```python
from build123d import *
from build123d.topology import SkipClean

# Parameters (mm, degrees)
SKETCH_1_W          = 101.5
SKETCH_1_H          = 91.5
SKETCH_1_W_2        = 98.5
SKETCH_1_H_2        = 88.5
EXTRUDE_1_DEPTH     = 21
SKETCH_2_W          = 101.5
SKETCH_2_H          = 91.5
SKETCH_2_R          = 1.5
SKETCH_2_W_2        = 31
SKETCH_2_H_2        = 31
EXTRUDE_2_DEPTH     = 1.5
SKETCH_3_R          = 1.75
CUT_EXTRUDE_1_DEPTH = 139.25881527
SKETCH_4_R          = 1.75
CUT_EXTRUDE_2_DEPTH = 139.25881527
FILLET_1_R          = 9
FILLET_2_R          = 10
FILLET_3_R          = 4
FILLET_4_R          = 5
EXTRUDE_START       = -3
SKETCH_5_R          = 47.5
SKETCH_5_R_2        = 1.5
SKETCH_5_W          = 45
SKETCH_5_H          = 46
EXTRUDE_3_DEPTH     = 3
SKETCH_6_R          = 47.5
SKETCH_6_R_2        = 43.5
EXTRUDE_4_DEPTH     = 13
SKETCH_7_R          = 49.25
SKETCH_7_R_2        = 43.5
EXTRUDE_5_DEPTH     = 9
SKETCH_8_R          = 44
SKETCH_8_R_2        = 5
CUT_EXTRUDE_3_DEPTH = 1.5
SKETCH_9_R          = 1.75
CUT_EXTRUDE_4_DEPTH = 141.599608819
SKETCH_10_R         = 3
CUT_EXTRUDE_5_DEPTH = 1.5


with BuildPart() as part:
    # 草图1 → 凸台-拉伸1 (new body)
    with BuildSketch(Plane(origin=(0, 0, 0), x_dir=(0, 0, -1), z_dir=(1, 0, 0))):
        with Locations((50.75, 45.75)):
            Rectangle(SKETCH_1_W, SKETCH_1_H)
        with Locations((50.75, 45.75)):
            Rectangle(SKETCH_1_W_2, SKETCH_1_H_2, mode=Mode.SUBTRACT)
    extrude(amount=EXTRUDE_1_DEPTH)

    # 草图2 → 凸台-拉伸2 (add)
    with BuildSketch(Plane.ZY):
        with Locations((-50.75, 45.75)):
            Rectangle(SKETCH_2_W, SKETCH_2_H)
        with Locations((-27.25, 71.5)):
            Circle(SKETCH_2_R, mode=Mode.SUBTRACT)
        with Locations((-22.25, 44.5)):
            Circle(SKETCH_2_R, mode=Mode.SUBTRACT)
        with Locations(Location((-79.25, 44.5, 0), (0, 0, 180))):
            Circle(SKETCH_2_R, mode=Mode.SUBTRACT)
        with Locations(Location((-74.25, 71.5, 0), (0, 0, 180))):
            Circle(SKETCH_2_R, mode=Mode.SUBTRACT)
        with Locations((-50.75, 45)):
            Rectangle(SKETCH_2_W_2, SKETCH_2_H_2, mode=Mode.SUBTRACT)
    extrude(amount=EXTRUDE_2_DEPTH)

    # 草图3 → 切除-拉伸1 (cut, through all)
    with BuildSketch(Plane.XY):
        with Locations((11, 45.75)):
            Circle(SKETCH_3_R)
    extrude(amount=-CUT_EXTRUDE_1_DEPTH, mode=Mode.SUBTRACT)

    # 草图4 → 切除-拉伸2 (cut, through all)
    with BuildSketch(Plane(origin=(0, 91.5, 0), x_dir=(1, 0, 0), z_dir=(0, 1, 0))):
        with Locations(Location((11, 16.75, 0), (0, 0, 270))):
            Circle(SKETCH_4_R)
        with Locations(Location((11, 84.75, 0), (0, 0, 90))):
            Circle(SKETCH_4_R)
    extrude(amount=-CUT_EXTRUDE_2_DEPTH, mode=Mode.SUBTRACT)

    # 圆角1
    fillet_1_edges = [part.edges().sort_by_distance(p)[0] for p in [
        (10.5, 90, -100),
        (10.5, 90, -1.5),
    ]]
    fillet(fillet_1_edges, radius=FILLET_1_R)

    # 圆角2
    fillet_2_edges = [part.edges().sort_by_distance(p)[0] for p in [
        (9.75, 91.5, 0),
        (9.75, 91.5, -101.5),
    ]]
    fillet(fillet_2_edges, radius=FILLET_2_R)

    # 圆角3
    fillet_3_edges = [part.edges().sort_by_distance(p)[0] for p in [
        (10.5, 1.5, -1.5),
        (10.5, 1.5, -100),
    ]]
    fillet(fillet_3_edges, radius=FILLET_3_R)

    # 圆角4
    fillet_4_edges = [part.edges().sort_by_distance(p)[0] for p in [
        (9.75, 0, -101.5),
        (9.75, 0, 0),
    ]]
    fillet(fillet_4_edges, radius=FILLET_4_R)

    # 草图5 → 凸台-拉伸3 (add)
    with BuildSketch(Plane.ZY.offset(1.5).offset(EXTRUDE_START)):
        with Locations((-50.75, 45.75)):
            Circle(SKETCH_5_R)
        with Locations((-27.25, 71.5)):
            Circle(SKETCH_5_R_2, mode=Mode.SUBTRACT)
        with Locations((-22.25, 44.5)):
            Circle(SKETCH_5_R_2, mode=Mode.SUBTRACT)
        with Locations(Location((-79.25, 44.5, 0), (0, 0, 180))):
            Circle(SKETCH_5_R_2, mode=Mode.SUBTRACT)
        with Locations(Location((-74.25, 71.5, 0), (0, 0, 180))):
            Circle(SKETCH_5_R_2, mode=Mode.SUBTRACT)
        with Locations((-50.75, 43)):
            Rectangle(SKETCH_5_W, SKETCH_5_H, mode=Mode.SUBTRACT)
    extrude(amount=EXTRUDE_3_DEPTH)

    # 草图6 → 凸台-拉伸4 (add)
    with BuildSketch(Plane(origin=(1.5, 0, 0), x_dir=(0, 0, -1), z_dir=(1, 0, 0))):
        with Locations(Location((50.75, 45.75, 0), (0, 0, 105.600995393))):
            Circle(SKETCH_6_R)
        with Locations((50.75, 45.75)):
            Circle(SKETCH_6_R_2, mode=Mode.SUBTRACT)
    extrude(amount=-EXTRUDE_4_DEPTH)

    # 草图7 → 凸台-拉伸5 (add)
    with BuildSketch(Plane.ZY.offset(11.5)):
        with Locations((-50.75, 45.75)):
            Circle(SKETCH_7_R)
        with Locations(Location((-50.75, 45.75, 0), (0, 0, 180))):
            Circle(SKETCH_7_R_2, mode=Mode.SUBTRACT)
    extrude(amount=EXTRUDE_5_DEPTH)

    # 草图8 → 切除-拉伸3 (cut)
    with BuildSketch(Plane(origin=(1.5, 0, 0), x_dir=(0, 0, -1), z_dir=(1, 0, 0))):
        with Locations((50.75, 45.75)):
            Circle(SKETCH_8_R)
        with Locations((74.25, 71.5)):
            Circle(SKETCH_8_R_2, mode=Mode.SUBTRACT)
        with Locations((79.25, 44.5)):
            Circle(SKETCH_8_R_2, mode=Mode.SUBTRACT)
        with Locations((22.25, 44.5)):
            Circle(SKETCH_8_R_2, mode=Mode.SUBTRACT)
        with Locations((27.25, 71.5)):
            Circle(SKETCH_8_R_2, mode=Mode.SUBTRACT)
    extrude(amount=-CUT_EXTRUDE_3_DEPTH, mode=Mode.SUBTRACT)

    # 草图9 → 切除-拉伸4 (cut, through all)
    with SkipClean():  # the faces are left unmerged after this step: merging them gives an invalid solid
        with BuildSketch(Plane.XY):
            with Locations((-6.5, 45.75)):
                Circle(SKETCH_9_R)
        extrude(amount=-CUT_EXTRUDE_4_DEPTH, mode=Mode.SUBTRACT)

    # 草图10 → 切除-拉伸5 (cut)
    with SkipClean():  # the faces are left unmerged after this step: merging them gives an invalid solid
        with BuildSketch(Plane.ZY.offset(1.5)):
            with Locations((-74.25, 71.5)):
                Circle(SKETCH_10_R)
            with Locations((-27.25, 71.5)):
                Circle(SKETCH_10_R)
            with Locations((-22.25, 44.5)):
                Circle(SKETCH_10_R)
            with Locations((-79.25, 44.5)):
                Circle(SKETCH_10_R)
        extrude(amount=-CUT_EXTRUDE_5_DEPTH, mode=Mode.SUBTRACT)


solid = part.part
```
Read the model definition and answer for the solid it produces. Units are mm, in the model's axes. A direction names the side the tool comes from. Give positions to 0.01 mm unless a question says otherwise; leave off trailing zeros. Write each loop counter-clockwise with the first axis right and the second up, starting at its lowest first coordinate (ties: lowest second). Pieces come first, ordered by that corner, then holes. Notation, with made-up numbers: (64.25, 5.5) -> (95.25, 5.5) arc R13 cw to (95.25, 30.5) -> close; hole circle Ø3 at (54, 6). An arc over 180 degrees is marked (long way). Answer as a JSON object with one key per item and string values.
1) Section A-A on z = -50.75 is taken. Write down the section's boundary in (x, y).
Findings below:
{"outline": "(-20.5, -3.5) -> (-11.5, -3.5) -> (-11.5, -1.75) -> (1.5, -1.75) -> (1.5, 0) -> (21, 0) -> (21, 1.5) -> (1.5, 1.5) -> (1.5, 1.75) -> (0, 1.75) -> (0, 29.5) -> (-1.5, 29.5) -> (-1.5, 2.25) -> (-20.5, 2.25) -> close; (-20.5, 89.25) -> (-1.5, 89.25) -> (-1.5, 60.5) -> (0, 60.5) -> (0, 89.75) -> (1.5, 89.75) -> (1.5, 90) -> (21, 90) -> (21, 91.5) -> (1.5, 91.5) -> (1.5, 93.25) -> (-11.5, 93.25) -> (-11.5, 95) -> (-20.5, 95) -> close"}
2) For a pull along Y with two mould halves and no side action, classify faces 1 (the cylindrical face through (-15.94, -2.33, -61.43)), 2 (the flat face through (10, 43, -101.5)), 3 (the flat face through (1.5, 73, -26)) as pulls with the +Y half, pulls with the -Y half, needs draft (parallel to the pull), parting line crosses it, or undercut.
Findings below:
{"face 1": "parting line crosses it", "face 2": "needs draft", "face 3": "undercut"}
3) Straight lines are drawn through the part: probe 1 along Y at (x, z) = (5.5, -45); probe 2 along Z at (x, y) = (4, 18.5); probe 3 along Y at (x, z) = (-7, -50). For each, find the intervals that lie inside material, in ascending order. Write a range as from..to.
Findings below:
{"probe 1": "y = 0..1.5, 90..91.5", "probe 2": "z = -101.5..-100, -1.5..0", "probe 3": "y = -1.74..2.26, 89.24..93.24"}
4) Section B-B on x = 15 is taken. Write down the section's boundary in (y, z), then the cut area to 3 significant figures.
Findings below:
{"outline": "(0, -96.5) arc R5 ccw to (5, -101.5) -> (81.5, -101.5) arc R10 ccw to (91.5, -91.5) -> (91.5, -10) arc R10 ccw to (81.5, 0) -> (5, 0) arc R5 ccw to (0, -5) -> close; hole (1.5, -96) arc R4 ccw to (5.5, -100) -> (81, -100) arc R9 ccw to (90, -91) -> (90, -10.5) arc R9 ccw to (81, -1.5) -> (5.5, -1.5) arc R4 ccw to (1.5, -5.5) -> close", "area": "558 mm^2"}
5) Flat-ended cylindrical pins translate along their axes: pin 1 Ø0.5 at (y, z) = (-1, -47) entering from +X; pin 2 Ø10 at (x, z) = (15, -73) entering from -Y; pin 3 Ø1.8 at (y, z) = (72, -26) entering from -X. Find the tip coordinate at first contact, or state that the pin passes through.
Findings below:
{"pin 1": "stops at x = 1.5", "pin 2": "stops at y = 0", "pin 3": "stops at x = 0"}
6) A tool of negligible diameter and unlimited length cuts with its end or side. For faces 4 (the flat face through (-1.5, 43, -2)), 5 (the flat face through (1.5, 43, -23)), 6 (the cylindrical face through (-6.353, 93.224, -52.307)), 7 (the cylindrical face through (10.474, 0.76, -86.419)), 8 (the cylindrical face through (-0.76, 46.53, -81.46)), from which of +Z, -Z, +X, -X, +Y, -Y can it reach the whole face along a straight path? Write none if from no direction.
Findings below:
{"face 4": "+Z", "face 5": "+X", "face 6": "none", "face 7": "+Y, -Y", "face 8": "-X"}
